Build history of the part. All positions in model axes, mm. Face numbers are marked on the shaded views. A direction names the side the tool comes from. Coordinates: 2 decimals unless noted, no trailing zeros. Write each loop counter-clockwise with the first axis right and the second up, starting at its lowest first coordinate (ties: lowest second). Pieces come first, ordered by that corner, then holes. Notation, with made-up numbers: (-27.75, -34) -> (6.25, -34) arc R9 ccw to (6.25, -29) -> close; hole circle Ø7 at (-23.75, -29). An arc over 180 degrees is marked (long way). Write each question's results on one line, items separated by ' | '. Start each with the question number.
Q1. Tool access for the marked faces 5, 6, 7, 8 and 9: list every direction of +Z, -Z, +X, -X, +Y, -Y with a clear straight run to the whole face (end or side of a thin tool).
Q2. Two-plate mould, pull along Z, no slides. Class the marked faces 1, 2, 3 and 4: released by +Z, released by -Z, zero draft, split by the parting line, or undercut.
Q3. Saw through at C-C on x = 32. Give the cut face in (y, z), and give its area (3 significant figures).
Q4. Drop flat-ended pins along their axis: pin 1 Ø10 at (x, z) = (7.5, 10) entering from +Y; pin 2 Ø7.5 at (y, z) = (11.5, 16) entering from +X; pin 3 Ø3.5 at (x, z) = (-12.5, 34.5) entering from -Y. Give the stop position or say it passes through.
Q5. Saw through at A-A on x = -7.5. Give the cut face in (y, z).
Q6. Drill centre lines: line 1 (X direction, y = 0.5, z = 7); line 2 (Z direction, x = -14, y = -6.75); line 3 (Z direction, x = 13.5, y = 12.5). Where is each one in solid material? Low to high.
Q7. Saw through at B-B on y = 0. Give the cut face in (x, z) (1 decimal).
Q8. Saw through at D-D on y = -8.5. Give the cut face in (x, z), and give its area (3 significant figures).
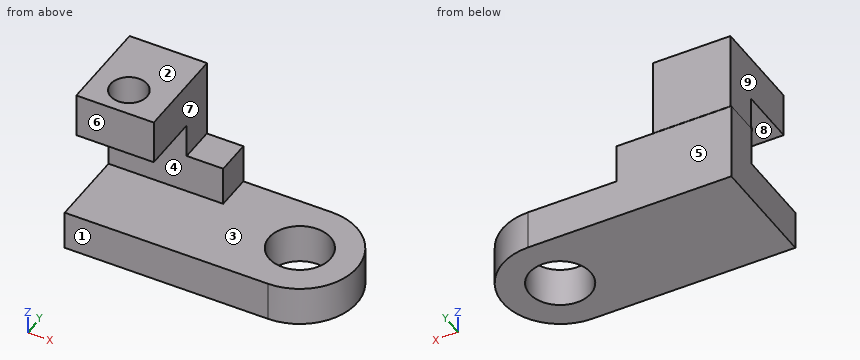
Autodesk Inventor part; units mm, degrees
ref_plane "YZ Plane" through (0, 0, 0) normal (1, 0, 0) x (0, 1, 0)
ref_plane "XZ Plane" through (0, 0, 0) normal (0, 1, 0) x (-1, 0, 0)
ref_plane "XY Plane" through (0, 0, 0) normal (0, 0, 1) x (1, 0, 0)
sketch "스케치1" plane through (0, 0, 0) normal (0, 0, 1) x (1, 0, 0)
  line L0 (25.8992, -14.5721) -> (-25.8992, -14.5721)
  line L1 (-25.8992, -14.5721) -> (-25.8992, 14.5721)
  line L2 (-25.8992, 14.5721) -> (25.8992, 14.5721)
  line L3 (25.8992, -14.5721) -> (-25.8992, 14.5721) construction
  line L4 (-25.8992, -14.5721) -> (25.8992, 14.5721) construction
  arc A0 (25.8992, -14.5721) -> (25.8992, 14.5721) centre (25.8992, 0) ccw
  circle A1 centre (25.8992, 0) radius 7.8142
  point P0 (0, 0)
extrude "돌출1" add sketch "스케치1" along normal blind 10
sketch "스케치2" plane through (0, 0, 10) normal (0, 0, 1) x (1, 0, 0)
  line L0 (-25.8992, 14.5721) -> (-25.8992, -14.5721)
  line L1 (-25.8992, 14.5721) -> (3.3382, 14.5721)
  line L2 (3.3382, 14.5721) -> (3.3382, 5.3954)
  line L3 (3.3382, 5.3954) -> (-25.8992, 5.3954)
  line L4 (-25.8992, 5.3954) -> (-25.8992, 14.5721)
  point P0 (0, 0)
extrude "돌출2" add sketch "스케치2" along normal blind 10
sketch "스케치3" plane through (0, 0, 20) normal (0, 0, 1) x (1, 0, 0)
  line L0 (-25.8992, 5.3954) -> (3.3382, 5.3954)
  line L1 (-25.7105, 14.6501) -> (-5.9667, 14.6501)
  line L2 (-5.9667, 14.6501) -> (-5.9667, 5.3954)
  line L3 (-5.9667, 5.3954) -> (-25.7105, 5.3954)
  line L4 (-25.7105, 5.3954) -> (-25.7105, 14.6501)
  point P0 (0, 0)
extrude "돌출3" add sketch "스케치3" along normal blind 20
sketch "스케치4" plane through (-25.8992, 5.3954, 10) normal (0, -1, 0) x (1, 0, 0)
  line L0 (0.1887, 30) -> (19.9325, 30)
  line L1 (19.9325, 10) -> (19.9325, 30)
  line L2 (0.1887, 30) -> (19.9325, 30)
  line L3 (19.9325, 30) -> (19.9325, 18.6928)
  line L4 (19.9325, 18.6928) -> (0.1887, 18.6928)
  line L5 (0.1887, 18.6928) -> (0.1887, 30)
  point P0 (25.8992, -10)
extrude "돌출4" add sketch "스케치4" along normal blind 15
sketch "스케치5" plane through (0, 0, 40) normal (0, 0, 1) x (1, 0, 0)
  circle A0 centre (-16.4269, -2.2401) radius 4.6425
  point P0 (0, 0)
extrude "돌출5" cut sketch "스케치5" against normal blind 15
properties part number "240503_3Dsketch07"
Returned:
1) face 5: -Z, +X, -X, +Y | face 6: +Z, +X, -X, -Y | face 7: +Z, +X, +Y, -Y | face 8: +X, -X, -Y | face 9: +Z, -X, +Y, -Y
2) face 1: zero draft | face 2: released by +Z | face 3: undercut | face 4: undercut
3) outline: (-13.23, 0) -> (-4.88, 0) -> (-4.88, 10) -> (-13.23, 10) -> close; (4.88, 0) -> (13.23, 0) -> (13.23, 10) -> (4.88, 10) -> close | area: 167 mm2
4) pin 1: stops at y = 14.57 | pin 2: stops at x = 3.34 | pin 3: stops at y = -9.6
5) outline: (-14.57, 0) -> (14.57, 0) -> (14.57, 20) -> (14.65, 20) -> (14.65, 40) -> (-9.6, 40) -> (-9.6, 28.69) -> (5.4, 28.69) -> (5.4, 10) -> (-14.57, 10) -> close
6) line 1: x = -25.9 to 18.1, 33.7 to 40.46 | line 2: z = 0 to 10, 28.69 to 40 | line 3: z = 0 to 10
7) outline: (-25.9, 0) -> (18.1, 0) -> (18.1, 10) -> (-25.9, 10) -> close; (-25.7, 28.7) -> (-20.5, 28.7) -> (-20.5, 40) -> (-25.7, 40) -> close; (-12.4, 28.7) -> (-6, 28.7) -> (-6, 40) -> (-12.4, 40) -> close; (33.7, 0) -> (40.5, 0) -> (40.5, 10) -> (33.7, 10) -> close
8) outline: (-25.9, 0) -> (37.74, 0) -> (37.74, 10) -> (-25.9, 10) -> close; (-25.71, 28.69) -> (-5.97, 28.69) -> (-5.97, 40) -> (-25.71, 40) -> close | area: 860 mm2
